Autodesk Inventor part; units mm, degrees
ref_plane "YZ Plane" through (0, 0, 0) normal (1, 0, 0) x (0, 1, 0)
ref_plane "XZ Plane" through (0, 0, 0) normal (0, 1, 0) x (-1, 0, 0)
ref_plane "XY Plane" through (0, 0, 0) normal (0, 0, 1) x (1, 0, 0)
sketch "Sketch1" plane through (0, 0, 0) normal (0, 1, 0) x (-1, 0, 0)
  line L0 (-2.5, 0) -> (-2.5, 10.795)
  line L1 (-2.5, 10.795) -> (-6.35, 10.795)
  line L2 (-6.35, 10.795) -> (-6.35, 4.445)
  arc A0 (-6.35, 1.905) -> (-6.35, 4.445) centre (-6.7204, 3.175) ccw
  line L3 (-6.35, 1.905) -> (-6.35, 0)
  line L4 (-6.35, 0) -> (-2.5, 0)
  line L5 (-6.7204, 3.175) -> (-5.3975, 3.175)
  line L6 (0, -2.159) -> (0, 12.954)
  point P0 (0, 0)
  dimension "d0" = 2.5
  dimension "d1" = 6.35
  dimension "d2" = 5.3975
  dimension "d3" = 10.795
  dimension "d4" = 7.62
  dimension "d5" = 2.54
revolve "Revolution1" add sketch "Sketch1" angle 360 about axis through (0, 0, -10) along (0, 0, 1)
properties part number "HOBBED PULLEY"
Verification items for the finished model (mm, model axes). Give positions to 0.01 mm unless a question says otherwise; leave off trailing zeros. Order: outer loops, then holes, each group sorted by start corner. A loop starts at its lowest first (then second) coordinate and runs counter-clockwise, first axis right, second up. Notation, with made-up numbers: M -11.75,3 L 30.25,3 A22 ccw 30.25,28 Z; hole C 21,70.5 d6. An arc over 180 degrees is marked long. Return JSON: item names as keys, results as strings. Group by question number.
1) Mould release check, pull along X, two halves, no side actions. Record for faces 1 (the face through (3, 0, 0)), 2 (the face through (-1.38, 6.2, 0.94)), 3 (the face through (-0.54, -2.44, 5.47)): pulls with the +X half, pulls with the -X half, needs draft (parallel to the pull), parting line crosses it, or undercut.
2) Go/stop test with flat-tipped pins: pin 1 Ø1 at (x, z) = (-2.5, 2) entering from -Y; pin 2 Ø1 at (x, z) = (5, 8) entering from +Y; pin 3 Ø1.5 at (x, z) = (-3.5, 1) entering from -Y. Record where each tip stops, or that it passes through.
3) Section check A-A on x = 0. Record the cut outline in (y, z) (3 decimals), and give its area (3 significant figures).
4) Scan lines: line 1 (Y direction, x = 0, z = 5.75); line 2 (Y direction, x = 0, z = 3); line 3 (Z direction, x = 4.25, y = 4) (3 decimals). Record each from-to range of solid material in increasing order.
5) Section check C-C on z = 8.5. Record the cut outline in (x, y), and give its area (3 significant figures).
Answer block:
{
 "1": {"face 1": "needs draft", "face 2": "parting line crosses it", "face 3": "undercut"},
 "2": {"pin 1": "stops at y = -6.02", "pin 2": "stops at y = 4.48", "pin 3": "stops at y = -5.72"},
 "3": {"outline": "M -6.35,0 L -2.5,0 L -2.5,10.795 L -6.35,10.795 L -6.35,4.445 A1.323 cw -6.35,1.905 Z; M 2.5,0 L 6.35,0 L 6.35,1.905 A1.323 cw 6.35,4.445 L 6.35,10.795 L 2.5,10.795 Z", "area": "79.6 mm^2"},
 "4": {"line 1": "y = -6.35 to -2.5, 2.5 to 6.35", "line 2": "y = -5.41 to -2.5, 2.5 to 5.41", "line 3": "z = 0 to 2.191, 4.159 to 10.795"},
 "5": {"outline": "C 0,0 d12.7; hole C 0,0 d5", "area": "107 mm^2"}
}
